Verification items for the finished model (mm, model axes). Face numbers are marked on the shaded views. A direction names the side the tool comes from. Round coordinates to 2 decimals unless told otherwise and drop trailing zeros. Write each loop counter-clockwise with the first axis right and the second up, starting at its lowest first coordinate (ties: lowest second). Pieces come first, ordered by that corner, then holes. Notation, with made-up numbers: M -35.75,48.25 L -20.75,48.25 A15 ccw -20.75,59.25 Z; hole C 47,61 d4. An arc over 180 degrees is marked long. Answer in a Markdown table with one row per item. Add a question column.
1. Draft check along X on the marked faces 4 and 5. Enter one of: pulls with the +X half, pulls with the -X half, needs draft (parallel to the pull), parting line crosses it, or undercut.
2. Sectioned sample at C-C on x = -7.25. Record the cut outline in (y, z).
3. Set-up check for the marked faces 1, 2 and 3: record each of +Z, -Z, +X, -X, +Y, -Y from which the full face is reachable in a straight line by a thin tool's end or side.
4. Go/stop test with flat-tipped pins: pin 1 Ø1.5 at (y, z) = (0, 0.5) entering from -X; pin 2 Ø1.3 at (x, y) = (-6, -0.5) entering from +Z; pin 3 Ø0.7 at (x, y) = (-4, 0) entering from +Z. Record where each tip stops, or that it passes through.
5. Sectioned sample at B-B on z = 5. Record the cut outline in (x, y), plus the area to 3 significant figures.
6. Sectioned sample at A-A on y = -0.15. Record the cut outline in (x, z), plus the area to 3 significant figures.
7. Material ranges on probe 1 along X at (y, z) = (-0.15, 1); probe 2 along Y at (x, z) = (-2.5, 6.5); probe 3 along Z at (x, y) = (-13.5, 0.15), recorded low to high.
Autodesk Inventor part; units mm, degrees
ref_plane "Work Plane1" through (-5.4042, -0.3175, 7.6401) normal (-1, 0, 0) x (0, 0, 1)
ref_plane "YZ Plane" through (0, 0, 0) normal (1, 0, 0) x (0, 1, 0)
ref_plane "XZ Plane" through (0, 0, 0) normal (0, 1, 0) x (-1, 0, 0)
sketch "Sketch1" plane through (0, 0, 0) normal (0, 1, 0) x (-1, 0, 0)
  line L0 (2.5467, 7.6401) -> (1.9117, 7.6401)
  line L1 (1.9117, 7.6401) -> (1.9117, -1.0276)
  line L2 (2.7055, -1.8214) -> (14.6752, -1.8214)
  line L3 (14.6752, -1.8214) -> (14.6752, -1.1864)
  line L4 (14.6752, -1.1864) -> (3.3405, -1.1864)
  line L5 (2.5467, 7.6401) -> (2.5467, -0.3926)
  line L6 (14.6752, -1.5039) -> (20.4389, -1.5039) construction
  line L7 (2.2292, 7.6401) -> (2.2292, 18.3973) construction
  line L8 (8.8332, 0.2741) -> (6.2932, 0.2741) construction
  line L9 (6.2932, 0.2741) -> (6.2932, -2.8247) construction
  line L10 (8.8332, -2.8247) -> (8.8332, 0.2741) construction
  arc A0 (2.5467, -0.3926) -> (3.3405, -1.1864) centre (3.3405, -0.3926) ccw
  arc A1 (1.9117, -1.0276) -> (2.7055, -1.8214) centre (2.7055, -1.0276) ccw
  line L11 (8.8332, -2.8247) -> (6.2932, -2.8247) construction
  dimension "d2" = 0.635
  dimension "d7" = 3.0988
  dimension "d9" = 1.778
  dimension "d10" = 7.366
  dimension "d11" = 4.064
  dimension "d12" = 5.842
  dimension "d13" = 0.7937
extrude "Extrusion1" add sketch "Sketch1" along normal mid plane 0.635
ref_plane "Work Plane1" through (-5.4042, -0.3175, 7.6401) normal (-1, 0, 0) x (0, 0, 1)
sketch "Sketch2" plane through (-5.4042, -0.3175, 7.6401) normal (-1, 0, 0) x (0, 0, 1)
  line L0 (-8.8265, 0) -> (-8.8265, 0.635)
  line L1 (-9.4615, 0.635) -> (-8.8265, 0.635)
  line L2 (-9.4615, 0) -> (-9.4615, 0.635)
  line L3 (-8.8265, 0) -> (-9.4615, 0)
  line L4 (-7.0485, -0.9525) -> (-10.1473, -0.9525)
  line L5 (-10.1473, -0.9525) -> (-10.1473, 1.5875)
  line L6 (-10.1473, 1.5875) -> (-7.0485, 1.5875)
  line L7 (-7.0485, 1.5875) -> (-7.0485, -0.9525)
  line L8 (-9.144, 0) -> (-9.144, -1.4837) construction
  line L9 (-11.684, 0) -> (-11.684, -1.596) construction
  line L10 (-14.224, 0) -> (-14.224, -1.596) construction
  line L11 (-9.4615, 0.3175) -> (-12.8271, 0.3175) construction
  point P0 (-7.6401, 0.3175)
  point P1 (-10.1473, 0.3175)
  dimension "d17" = 3.0988
  dimension "d18" = 1.778
  dimension "d19" = 2.54
extrude "Extrusion2" add sketch "Sketch2" along normal blind 2.54
properties part number "HeaderRight1"
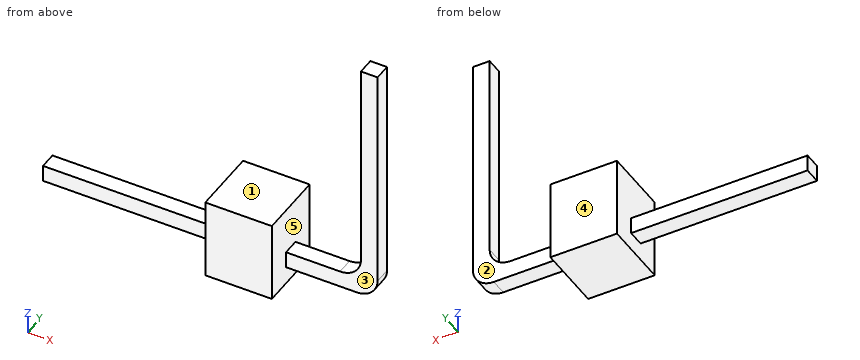
Geometry check:
| question | item | result |
|---|---|---|
| 1 | face 4 | needs draft |
| 1 | face 5 | undercut |
| 2 | outline | M -1.27,-2.51 L 1.27,-2.51 L 1.27,0.59 L -1.27,0.59 Z |
| 3 | face 1 | +Z, -X, +Y, -Y |
| 3 | face 2 | +Z, -Z, +X, +Y |
| 3 | face 3 | +Z, -Z, +X, -Y |
| 4 | pin 1 | stops at x = -7.94 |
| 4 | pin 2 | stops at z = 0.59 |
| 4 | pin 3 | stops at z = -1.19 |
| 5 | outline | M -2.55,-0.32 L -1.91,-0.32 L -1.91,0.32 L -2.55,0.32 Z |
| 5 | area | 0.403 mm2 |
| 6 | outline | M -14.68,-1.82 L -7.94,-1.82 L -7.94,-2.51 L -5.4,-2.51 L -5.4,-1.82 L -2.71,-1.82 A0.79 ccw -1.91,-1.03 L -1.91,7.64 L -2.55,7.64 L -2.55,-0.39 A0.79 cw -3.34,-1.19 L -5.4,-1.19 L -5.4,0.59 L -7.94,0.59 L -7.94,-1.19 L -14.68,-1.19 Z |
| 6 | area | 20.0 mm2 |
| 7 | probe 1 | x = -2.55 to -1.91 |
| 7 | probe 2 | y = -0.32 to 0.32 |
| 7 | probe 3 | z = -1.82 to -1.19 |
